from build123d import *

# Parameters (mm, degrees)
SKETCH_1_R          = 7
SKETCH_1_R_2        = 1.65
EXTRUDE_1_DEPTH     = 1
SKETCH_1_4_R        = 6
SKETCH_1_4_R_2      = 1.65
EXTRUDE_2_DEPTH     = 1.5
SKETCH_1_5_R        = 5
SKETCH_1_5_R_2      = 1.65
EXTRUDE_3_DEPTH     = 12
EXTRUDE_START       = 2
SKETCH_1_6_R        = 5
SKETCH_1_6_R_2      = 4.25
EXTRUDE_4_DEPTH     = 10
SKETCH_1_7_W        = 5.5
SKETCH_1_7_H        = 5.5
SKETCH_1_7_R        = 1.65
EXTRUDE_5_DEPTH     = 13
SKETCH_1_8_R        = 1.65
EXTRUDE_6_DEPTH     = 2
SKETCH_2_R          = 1
CUT_EXTRUDE_1_DEPTH = 2
FILLET_1_R          = 1
CHAMFER_1_SIZE      = 0.2
CHAMFER_2_SIZE      = 0.3


with BuildPart() as part:
    # Sketch 1 → Extrude 1 (new body)
    with BuildSketch(Plane(origin=(0, 0, 0), x_dir=(1, 0, 0), z_dir=(0, 1, 0))):
        with Locations(Location((0, 0, 0), (0, 0, 270))):
            Circle(SKETCH_1_R)
        with Locations(Location((0, 0, 0), (0, 0, 270))):
            Circle(SKETCH_1_R_2, mode=Mode.SUBTRACT)
    extrude(amount=EXTRUDE_1_DEPTH)

    # Sketch 1_4 → Extrude 2 (add)
    with BuildSketch(Plane(origin=(0, 0, 0), x_dir=(1, 0, 0), z_dir=(0, 1, 0))):
        with Locations(Location((0, 0, 0), (0, 0, 270))):
            Circle(SKETCH_1_4_R)
        with Locations(Location((0, 0, 0), (0, 0, 270))):
            Circle(SKETCH_1_4_R_2, mode=Mode.SUBTRACT)
    extrude(amount=EXTRUDE_2_DEPTH)

    # Sketch 1_5 → Extrude 3 (add)
    with BuildSketch(Plane(origin=(0, 0, 0), x_dir=(1, 0, 0), z_dir=(0, 1, 0))):
        with Locations(Location((0, 0, 0), (0, 0, 270))):
            Circle(SKETCH_1_5_R)
        with Locations(Location((0, 0, 0), (0, 0, 270))):
            Circle(SKETCH_1_5_R_2, mode=Mode.SUBTRACT)
    extrude(amount=EXTRUDE_3_DEPTH)

    # Sketch 1_6 → Extrude 4 (add)
    with BuildSketch(Plane(origin=(0, 0, 0), x_dir=(1, 0, 0), z_dir=(0, 1, 0)).offset(EXTRUDE_START)):
        with Locations(Location((0, 0, 0), (0, 0, 270))):
            Circle(SKETCH_1_6_R)
        Circle(SKETCH_1_6_R_2, mode=Mode.SUBTRACT)
    extrude(amount=EXTRUDE_4_DEPTH)

    # Sketch 1_7 → Extrude 5 (add)
    with BuildSketch(Plane(origin=(0, 0, 0), x_dir=(1, 0, 0), z_dir=(0, 1, 0)).offset(EXTRUDE_START)):
        Rectangle(SKETCH_1_7_W, SKETCH_1_7_H)
        with Locations(Location((0, 0, 0), (0, 0, 270))):
            Circle(SKETCH_1_7_R, mode=Mode.SUBTRACT)
    extrude(amount=EXTRUDE_5_DEPTH)

    # Sketch 1_8 → Extrude 6 (add)
    with BuildSketch(Plane(origin=(0, 0, 0), x_dir=(1, 0, 0), z_dir=(0, 1, 0))):
        with Locations(Location((0, 0, 0), (0, 0, 270))):
            Circle(SKETCH_1_8_R)
    extrude(amount=EXTRUDE_6_DEPTH)

    # Sketch 2 → Cut-Extrude 1 (cut)
    with BuildSketch(Plane.XZ):
        with Locations((0, -3)):
            Circle(SKETCH_2_R)
        with BuildLine():
            Line((-1, 3), (-1, -3))
            ThreePointArc((-1, -3), (0, -2), (1, -3))
            Line((1, -3), (1, 3))
            ThreePointArc((1, 3), (0, 2), (-1, 3))
        make_face()
        with Locations((0, 3)):
            Circle(SKETCH_2_R)
    extrude(amount=-CUT_EXTRUDE_1_DEPTH, mode=Mode.SUBTRACT)

    # Fillet 1
    fillet_1_edges = [part.edges().sort_by_distance(p)[0] for p in [
        (-2.75, 13.5, 2.75),
        (2.75, 13.5, 2.75),
        (2.75, 13.5, -2.75),
        (-2.75, 13.5, -2.75),
    ]]
    fillet(fillet_1_edges, radius=FILLET_1_R)

    # Chamfer 1
    chamfer_1_edges = [part.edges().sort_by_distance(p)[0] for p in [
        (0, 12, -5),
        (0, 0, -7),
        (0, 15, -1.65),
        (0, 1, -7),
    ]]
    chamfer(chamfer_1_edges, length=CHAMFER_1_SIZE)

    # Chamfer 2
    chamfer_2_edges = [part.edges().sort_by_distance(p)[0] for p in [
        (2.75, 15, 0),
        (0, 15, 2.75),
        (0, 15, -2.75),
        (-2.75, 15, 0),
        (-2.457106781, 15, 2.457106781),
        (-2.457106781, 15, -2.457106781),
        (2.457106781, 15, -2.457106781),
        (2.457106781, 15, 2.457106781),
    ]]
    chamfer(chamfer_2_edges, length=CHAMFER_2_SIZE)

    # Sketch 3 → Cut-Revolve 1 (revolve, cut)
    with BuildSketch(Plane(origin=(0, 0, 0), x_dir=(0, 0, -1), z_dir=(1, 0, 0)), mode=Mode.PRIVATE) as cut_revolve_1_sk:
        Polygon((0, 2), (0, 1.316547622), (-1.65, 2), align=None)
    revolve(cut_revolve_1_sk.sketch.rotate(Axis((0, 11.8, 0), (0, -1, 0)), 217.305200966), axis=Axis((0, 11.8, 0), (0, -1, 0)), mode=Mode.SUBTRACT)


solid = part.part
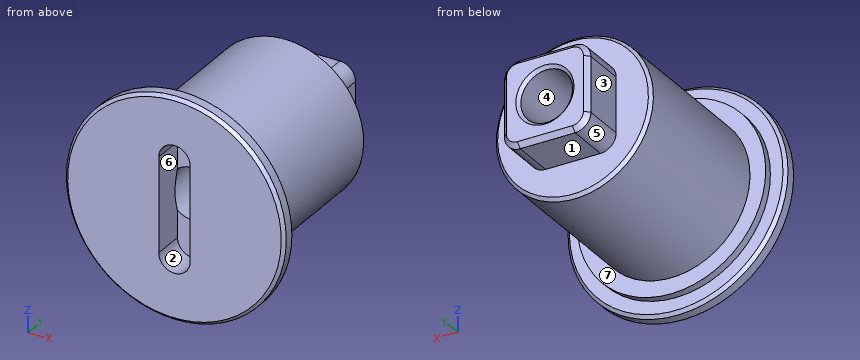
Geometry check sheet. Reference: the model listing, model coordinates, mm. Face numbers are marked on the shaded views. A direction names the side the tool comes from. Round coordinates to 2 decimals unless told otherwise and drop trailing zeros. Order: outer loops, then holes, each group sorted by start corner. A loop starts at its lowest first (then second) coordinate and runs counter-clockwise, first axis right, second up. Notation, with made-up numbers: M -18,36.25 L 22,36.25 A8 cw 22,47.25 Z; hole C 83.5,67.25 d1. An arc over 180 degrees is marked long. Answer in a Markdown table with one row per item.
(1) Scan lines: probe 1 along X at (y, z) = (13.5, 0); probe 2 along X at (y, z) = (9.25, 0); probe 3 along Y at (x, z) = (-5.75, 2.25). Record each from-to range of solid material in increasing order. Write a range as from..to.
Responses:
| item | result |
|---|---|
| probe 1 | x = -2.75..-1.65, 1.65..2.75 |
| probe 2 | x = -5..-1.65, 1.65..5 |
| probe 3 | y = 0..1 |
(2) Draft check along X on the marked faces 5, 6 and 7. Enter one of: released by +X, released by -X, zero draft, split by the parting line, or undercut.
Responses:
| item | result |
|---|---|
| face 5 | released by -X |
| face 6 | undercut |
| face 7 | zero draft |
(3) Tool access check on the marked faces 1, 2, 3 and 4. Record the directions out of +Z, -Z, +X, -X, +Y, -Y that give a thin tool (end or side, any length) a straight path to the whole face; none if there is none.
Responses:
| item | result |
|---|---|
| face 1 | -Z, +X, -X, +Y |
| face 2 | -Y |
| face 3 | +Z, -Z, -X, +Y |
| face 4 | +Y |
(4) Go/stop test with flat-tipped pins: P1, Ø1.6, axis at y = 1, z = 1, coming from the -X side; P2, Ø1, axis at y = 1, z = -0.5, coming from the +X side; P3, Ø0.6, axis at x = 0, z = -2.5, coming from the -Y side; P4, Ø3, axis at x = 3.5, y = 7.5, coming from the +Z side. Record where each tip stops, or that it passes through.
Responses:
| item | result |
|---|---|
| P1 | stops at x = -7 |
| P2 | stops at x = 7 |
| P3 | stops at y = 2 |
| P4 | stops at z = 4.58 |
(5) Sectioned sample at C-C, the plane y = 8.5. Record the cut outline in (x, z), and give its area (3 significant figures).
Responses:
| item | result |
|---|---|
| outline | C 0,0 d10; hole C 0,0 d3.3 |
| area | 70.0 mm² |
